Could you check a few things on this model? Use its own coordinates, in mm. A direction names the side the tool comes from. Coordinates: 2 decimals unless noted, no trailing zeros. Write each loop counter-clockwise with the first axis right and the second up, starting at its lowest first coordinate (ties: lowest second). Pieces come first, ordered by that corner, then holes. Notation, with made-up numbers: M 70,-7 L 126,-7 A21 cw 126,28 Z; hole C -17.5,-5.75 d1. An arc over 180 degrees is marked long. Write item = value, one per line.
```python
from build123d import *

# Parameters (mm, degrees)
BOSS_EXTRUDE1_DEPTH              = 330.200001
BOSS_EXTRUDE1_DEPTH_BACK         = 330.200001
SKETCH3_W                        = 50.8
SKETCH3_H                        = 25.4
SKETCH3_W_2                      = 44.45
SKETCH3_H_2                      = 19.05
F_1_4_0_25_DIAMETER_HOLE3_D      = 6.35
F_1_4_0_25_DIAMETER_HOLE4_D      = 6.35
F_1_4_0_25_DIAMETER_HOLE5_D      = 6.35
F_1_4_0_25_DIAMETER_HOLE6_D      = 6.35
F_1_4_0_25_DIAMETER_HOLE7_D      = 6.35
F_1_4_0_25_DIAMETER_HOLE8_D      = 6.35
F_13_64_0_20313_DIAMETER_HOLE1_D = 5.159502
F_1_2_0_5_DIAMETER_HOLE1_D       = 12.7
F_1_2_0_5_DIAMETER_HOLE1_DEPTH   = 6.35
F_1_2_0_5_DIAMETER_HOLE1_TIP     = 3.815464931
F_10_CLEARANCE_HOLE1_AT_2_COUNT  = 2
F_10_CLEARANCE_HOLE1_AT_2_PITCH  = 26.179508771
F_10_CLEARANCE_HOLE1_AT_3_COUNT  = 2
F_10_CLEARANCE_HOLE1_AT_3_PITCH  = 32.162957462
F_10_CLEARANCE_HOLE1_AT_4_COUNT  = 2
F_10_CLEARANCE_HOLE1_AT_4_PITCH  = 33.11362798
SKETCH35_R                       = 14.2875
CUT_EXTRUDE1_DEPTH               = 333.148100492
TAP_DRILL_FOR_8_32_TAP1_D        = 3.4544
F_1_4_0_25_DIAMETER_HOLE9_D      = 6.35
F_1_4_0_25_DIAMETER_HOLE10_D     = 6.35
F_1_4_0_25_DIAMETER_HOLE10_DEPTH = 5.08
F_1_4_0_25_DIAMETER_HOLE10_TIP   = 1.907732465


with BuildPart() as part:
    # Sketch3 → Boss-Extrude1 (new, two sides: drawn at the far end of the back side and taken through both)
    with BuildSketch(Plane.XY.offset(-BOSS_EXTRUDE1_DEPTH_BACK)):
        Rectangle(SKETCH3_W, SKETCH3_H)
        Rectangle(SKETCH3_W_2, SKETCH3_H_2, mode=Mode.SUBTRACT)
    extrude(amount=BOSS_EXTRUDE1_DEPTH + BOSS_EXTRUDE1_DEPTH_BACK)

    # 1/4 (0.25) Diameter Hole3 (through all)
    with Locations(Plane.ZY.offset(25.4)):
        with Locations((-317.500000508, 0)):
            Hole(F_1_4_0_25_DIAMETER_HOLE3_D / 2)

    # 1/4 (0.25) Diameter Hole4 (through all)
    with Locations(Plane.ZY.offset(25.4)):
        with Locations((292.100000508, 0), (317.500000508, 0)):
            Hole(F_1_4_0_25_DIAMETER_HOLE4_D / 2)

    # 1/4 (0.25) Diameter Hole5 (through all)
    with Locations(Plane(origin=(25.4, 0, 0), x_dir=(0, 0, -1), z_dir=(1, 0, 0))):
        with Locations((292.100000508, 0), (266.700000508, 0)):
            Hole(F_1_4_0_25_DIAMETER_HOLE5_D / 2)

    # 1/4 (0.25) Diameter Hole6 (through all)
    with Locations(Plane(origin=(25.4, 0, 0), x_dir=(0, 0, -1), z_dir=(1, 0, 0))):
        with Locations((215.900000508, 0), (241.300000508, 0)):
            Hole(F_1_4_0_25_DIAMETER_HOLE6_D / 2)

    # 1/4 (0.25) Diameter Hole7 (through all)
    with Locations(Plane(origin=(25.4, 0, 0), x_dir=(0, 0, -1), z_dir=(1, 0, 0))):
        with Locations((-190.5, 0), (-215.9, 0)):
            Hole(F_1_4_0_25_DIAMETER_HOLE7_D / 2)

    # 1/4 (0.25) Diameter Hole8 (through all)
    with Locations(Plane(origin=(25.4, 0, 0), x_dir=(0, 0, -1), z_dir=(1, 0, 0))):
        with Locations((-266.7, 0), (-241.3, 0)):
            Hole(F_1_4_0_25_DIAMETER_HOLE8_D / 2)

    # 13/64 (0.20313) Diameter Hole1 (through all)
    with Locations(Plane(origin=(25.4, 0, 0), x_dir=(0, 0, -1), z_dir=(1, 0, 0))):
        with Locations((-152.4, 0), (177.8, 0)):
            Hole(F_13_64_0_20313_DIAMETER_HOLE1_D / 2)

    # 1/2 (0.5) Diameter Hole1
    with Locations(Plane.ZY.offset(25.4)):
        with Locations((-591.301639708, -480.802221962), (-103.1875, 0), (77.7875, 0), (103.1875, 0), (-128.5875, 0)):
            Hole(F_1_2_0_5_DIAMETER_HOLE1_D / 2, depth=F_1_2_0_5_DIAMETER_HOLE1_DEPTH)
            with Locations((0, 0, -(F_1_2_0_5_DIAMETER_HOLE1_DEPTH + F_1_2_0_5_DIAMETER_HOLE1_TIP / 2))):  # 118° drill point
                Cone(0, F_1_2_0_5_DIAMETER_HOLE1_D / 2, F_1_2_0_5_DIAMETER_HOLE1_TIP, mode=Mode.SUBTRACT)

    # Sketch34 → #10 Clearance Hole1 (revolve, cut)
    with BuildSketch(Plane(origin=(-13.81901292, -12.7, -143.631885069), x_dir=(0, 0, -1), z_dir=(1, 0, 0))):
        Polygon((0, 0), (0, 25.4), (5.2197, 25.4), (2.4892, 22.258919064), (2.4892, 0), align=None)
    f_10_clearance_hole1 = revolve(axis=Axis((-13.81901292, -19.05, -143.631885069), (0, 1, 0)), mode=Mode.SUBTRACT)

    # #10 Clearance Hole1 at 2: #10 Clearance Hole1 ×2
    with Locations(*[Vector(-0.15706842311694033, 0, 0.9875877229186063) * (i * F_10_CLEARANCE_HOLE1_AT_2_PITCH) for i in range(1, F_10_CLEARANCE_HOLE1_AT_2_COUNT)]):
        add(f_10_clearance_hole1, mode=Mode.SUBTRACT)

    # #10 Clearance Hole1 at 3: #10 Clearance Hole1 ×2
    with Locations(*[Vector(0.8593123276123446, 0, 0.5114511937745914) * (i * F_10_CLEARANCE_HOLE1_AT_3_PITCH) for i in range(1, F_10_CLEARANCE_HOLE1_AT_3_COUNT)]):
        add(f_10_clearance_hole1, mode=Mode.SUBTRACT)

    # #10 Clearance Hole1 at 4: #10 Clearance Hole1 ×2
    with Locations(*[Vector(0.9588197348681927, 0, -0.28401534470392387) * (i * F_10_CLEARANCE_HOLE1_AT_4_PITCH) for i in range(1, F_10_CLEARANCE_HOLE1_AT_4_COUNT)]):
        add(f_10_clearance_hole1, mode=Mode.SUBTRACT)

    # Sketch35 → Cut-Extrude1 (cut, through all)
    with BuildSketch(Plane.XZ.offset(12.7)):
        with Locations((-7.9375, -186.037603725)):
            Circle(SKETCH35_R)
    extrude(amount=-CUT_EXTRUDE1_DEPTH, mode=Mode.SUBTRACT)

    # Tap Drill for #8-32 Tap1 (through all)
    with Locations(Plane(origin=(0, -12.7, 0), x_dir=(-1, 0, 0), z_dir=(0, -1, 0))):
        with Locations((-4.814463692, 198.789567417)):
            Hole(TAP_DRILL_FOR_8_32_TAP1_D / 2)

    # 1/4 (0.25) Diameter Hole9 (through all)
    with Locations(Plane(origin=(0, -12.7, 0), x_dir=(-1, 0, 0), z_dir=(0, -1, 0))):
        with Locations((-15.875, -161.925), (0, -76.2), (0, 76.2)):
            Hole(F_1_4_0_25_DIAMETER_HOLE9_D / 2)

    # 1/4 (0.25) Diameter Hole10
    with Locations(Plane(origin=(25.4, 0, 0), x_dir=(0, 0, -1), z_dir=(1, 0, 0))):
        with Locations((95.25, -4.45)):
            Hole(F_1_4_0_25_DIAMETER_HOLE10_D / 2, depth=F_1_4_0_25_DIAMETER_HOLE10_DEPTH)
            with Locations((0, 0, -(F_1_4_0_25_DIAMETER_HOLE10_DEPTH + F_1_4_0_25_DIAMETER_HOLE10_TIP / 2))):  # 118° drill point
                Cone(0, F_1_4_0_25_DIAMETER_HOLE10_D / 2, F_1_4_0_25_DIAMETER_HOLE10_TIP, mode=Mode.SUBTRACT)


solid = part.part
```
Item 1: For faces 4 (the face through (-9.797, 11.09, -171.872)), 5 (the face through (-23.79, 1.91, 97.13)), 6 (the face through (0, 9.525, -5)), which set-ups out of +Z, -Z, +X, -X, +Y, -Y let a thin tool reach every point of the face, with its end or its side?
Numbers:
face_4 = +Y, -Y
face_5 = -X
face_6 = +Z, -Z
Item 2: Imagine slicing it at A-A (z = -34). Write out the boundary of the cut face in (x, y) (3 decimals).
Numbers:
outline = M -25.4,-12.7 L 25.4,-12.7 L 25.4,12.7 L -25.4,12.7 Z; hole M -22.225,-9.525 L 22.225,-9.525 L 22.225,9.525 L -22.225,9.525 Z
Item 3: If I drill on line 1 along X through (y, z) = (-3, 254.5) (3 decimals); line 2 along Y through (x, z) = (18.5, 222.5) (3 decimals); line 3 along Y through (x, z) = (24.3, -266.7) (3 decimals), over which ranges is the centre line in solid material (lowest first)?
Numbers:
line_1 = -25.4 to -22.225, 22.225 to 25.4
line_2 = -12.7 to -9.525, 9.525 to 12.7
line_3 = -12.7 to -3.175, 3.175 to 12.7
Item 4: I'm going to push flat-ended pins straight in: P1, Ø4.5, axis at x = 17.93, z = -153.04, coming from the +Y side; P2, Ø6.5, axis at x = 13.82, z = -127.18, coming from the +Y side. Where does each tip first touch, or does it pass through?
Numbers:
P1 = through
P2 = 10.44
Item 5: If we mould it in two halves opening along Y, with no side actions, what happens to faces 1 (the face through (0, 10, -330.2)), 2 (the face through (-22.225, 0, -5)), 3 (the face through (0, 12.7, -5))? For each: pulls with the +Y half, pulls with the -Y half, needs draft (parallel to the pull), parting line crosses it, or undercut.
Numbers:
face_1 = needs draft
face_2 = undercut
face_3 = pulls with the +Y half
